Verification items for the finished model (mm, model axes). Round coordinates to 2 decimals unless told otherwise and drop trailing zeros. Write each loop counter-clockwise with the first axis right and the second up, starting at its lowest first coordinate (ties: lowest second). Pieces come first, ordered by that corner, then holes.
from build123d import *

# Parameters (mm, degrees)
AUFSATZ_LINEAR_AUSTRAGEN1_DEPTH = 52
SCHNITT_LINEAR_AUSTRAGEN1_DEPTH = 1
VERRUNDUNG2_R                   = 0.4


with BuildPart() as part:
    # Skizze1 → Aufsatz-Linear austragen1 (new body)
    with BuildSketch(Plane.XY):
        with BuildLine():
            Line((-23.5, 0.6), (23.5, 0.6))
            ThreePointArc((23.5, 0.6), (24.1, 0), (23.5, -0.6))
            Line((23.5, -0.6), (-23.5, -0.6))
            ThreePointArc((-23.5, -0.6), (-24.1, 0), (-23.5, 0.6))
        make_face()
    extrude(amount=AUFSATZ_LINEAR_AUSTRAGEN1_DEPTH)

    # Skizze2 → Schnitt-Linear austragen1 (cut)
    with BuildSketch(Plane(origin=(0, 0.6, 0), x_dir=(1, 0, 0), z_dir=(0, 1, 0))):
        with BuildLine():
            Line((-21.5, -49.8), (21.5, -49.8))
            ThreePointArc((21.5, -49.8), (22, -50.3), (21.5, -50.8))
            Line((21.5, -50.8), (-21.5, -50.8))
            ThreePointArc((-21.5, -50.8), (-22, -50.3), (-21.5, -49.8))
        make_face()
    extrude(amount=-SCHNITT_LINEAR_AUSTRAGEN1_DEPTH, mode=Mode.SUBTRACT)

    # Verrundung2
    verrundung2_edges = [part.edges().sort_by_distance(p)[0] for p in [
        (-22, -0.4, 50.3),
        (0, -0.4, 49.8),
        (22, -0.4, 50.3),
        (0, -0.4, 50.8),
    ]]
    fillet(verrundung2_edges, radius=VERRUNDUNG2_R)


solid = part.part
Q1. Sectioned sample at A-A (y = 0.3). Enter the section's corners in (x, z), plus the area to 3 significant figures.
Recorded:
outline: (-24.02, 0) - (24.02, 0) - (24.02, 52) - (-24.02, 52) - close; hole (-21.5, 49.8) - (21.5, 49.8) arc R0.5 ccw to (21.5, 50.8) - (-21.5, 50.8) arc R0.5 ccw to start
area: 2,450 mm2
Q2. Material ranges on line 1 along Z through (x, y) = (2.5, 0.4); line 2 along Z through (x, y) = (-10, -0.35); line 3 along X through (y, z) = (0.05, 6), recorded low to high.
Recorded:
line 1: z = 0 to 49.8, 50.8 to 52
line 2: z = 0 to 50.01, 50.59 to 52
line 3: x = -24.1 to 24.1
Q3. Release check for a two-part mould opening along Z. For faces 1 (the flat face through (0, 0, 52)), 2 (the flat face through (0, 0, 0)), 3 (the flat face through (0, -0.6, 26)) record: released by +Z, released by -Z, zero draft, split by the parting line, or undercut.
Recorded:
face 1: released by +Z
face 2: released by -Z
face 3: zero draft
